CAD build for the part. Positions are in the model's coordinates, mm. Give positions to 0.01 mm unless a question says otherwise; leave off trailing zeros. Loops run counter-clockwise (first coordinate to the right, second up) from the corner with the lowest first, then second, coordinate; pieces in that order, holes last.
Item 1: Probe probe 1 along Z at (x, y) = (-34.5, 0.25); probe 2 along Z at (x, y) = (-27, 0.15); probe 3 along X at (y, z) = (0.3, -26.5). List the from-to ranges inside material, lowest first.
Item 2: Saw through at D-D on z = -15.5. Give the cut face in (x, y), plus the area to 3 significant figures.
Item 3: Saw through at C-C on y = 0.1. Give the number of separate pieces and of enclosed holes in the cut face, plus the area to 3 significant figures.
Item 4: Saw through at B-B on z = -51.5. Give the cut face in (x, y).
Item 5: Saw through at A-A on x = -28.5. Give the cut face in (y, z), plus the area to 3 significant figures.
Autodesk Inventor part; units mm, degrees
ref_plane "YZ Plane" through (0, 0, 0) normal (1, 0, 0) x (0, 1, 0)
ref_plane "XZ Plane" through (0, 0, 0) normal (0, 1, 0) x (-1, 0, 0)
ref_plane "XY Plane" through (0, 0, 0) normal (0, 0, 1) x (1, 0, 0)
sketch "Эскиз1" plane through (0, 0, 0) normal (0, 1, 0) x (-1, 0, 0)
  line L0 (42.275, -3.8) -> (42.275, -4.36)
  arc A0 (40.675, -5.96) -> (42.275, -4.36) centre (40.675, -4.36) ccw
  line L1 (40.675, -5.96) -> (34.325, -5.96)
  arc A1 (32.725, -4.36) -> (34.325, -5.96) centre (34.325, -4.36) ccw
  line L2 (32.725, -4.36) -> (32.725, -3.8)
  arc A2 (34.325, -2.2) -> (32.725, -3.8) centre (34.325, -3.8) ccw
  line L3 (34.325, -2.2) -> (40.675, -2.2)
  arc A3 (42.275, -3.8) -> (40.675, -2.2) centre (40.675, -3.8) ccw
  arc A4 (55.5, -76.631) -> (57.5, -74.631) centre (55.5, -74.631) ccw
  line L4 (55.5, -76.631) -> (19.5, -76.631)
  arc A5 (17.5, -74.631) -> (19.5, -76.631) centre (19.5, -74.631) ccw
  line L5 (17.5, -74.631) -> (17.5, -58.631)
  arc A6 (19.5, -56.631) -> (17.5, -58.631) centre (19.5, -58.631) ccw
  line L6 (19.5, -56.631) -> (55.5, -56.631)
  arc A7 (57.5, -58.631) -> (55.5, -56.631) centre (55.5, -58.631) ccw
  line L7 (57.5, -58.631) -> (57.5, -74.631)
  line L8 (77.5, -85.631) -> (75, -85.631)
  line L9 (75, -47.631) -> (77.5, -47.631)
  line L10 (75, -47.631) -> (75, 0)
  line L11 (75, 0) -> (0, 0)
  line L12 (0, -47.631) -> (0, 0)
  line L13 (-2.5, -47.631) -> (0, -47.631)
  line L14 (0, -85.631) -> (-2.5, -85.631)
  line L15 (0, -85.631) -> (0, -133.2619)
  line L16 (0, -133.2619) -> (75, -133.2619)
  line L17 (75, -85.631) -> (75, -133.2619)
  line L18 (-0.95, -70.631) -> (-2.5, -70.631)
  line L19 (-2.5, -85.631) -> (-2.5, -70.631)
  line L20 (-2.5, -62.631) -> (-2.5, -47.631)
  line L21 (-2.5, -62.631) -> (-0.95, -62.631)
  line L22 (-0.95, -62.631) -> (-0.95, -63.131)
  line L23 (-4.831, -63.131) -> (-0.95, -63.131)
  line L24 (-4.831, -70.131) -> (-0.95, -70.131)
  line L25 (-0.95, -70.131) -> (-0.95, -70.631)
  arc A8 (-4.831, -63.131) -> (-4.831, -70.131) centre (-4.831, -66.631) ccw
  line L26 (77.5, -70.631) -> (77.5, -85.631)
  line L27 (77.5, -70.631) -> (75.95, -70.631)
  line L28 (75.95, -70.631) -> (75.95, -70.131)
  line L29 (79.831, -70.131) -> (75.95, -70.131)
  arc A9 (79.831, -70.131) -> (79.831, -63.131) centre (79.831, -66.631) ccw
  line L30 (79.831, -63.131) -> (75.95, -63.131)
  line L31 (75.95, -63.131) -> (75.95, -62.631)
  line L32 (75.95, -62.631) -> (77.5, -62.631)
  line L33 (77.5, -47.631) -> (77.5, -62.631)
  arc A10 (55.5, -76.631) -> (57.5, -74.631) centre (55.5, -74.631) ccw
  line L34 (57.5, -74.631) -> (57.5, -58.631)
  arc A11 (57.5, -58.631) -> (55.5, -56.631) centre (55.5, -58.631) ccw
  line L35 (55.5, -56.631) -> (19.5, -56.631)
  arc A12 (19.5, -56.631) -> (17.5, -58.631) centre (19.5, -58.631) ccw
  line L36 (17.5, -58.631) -> (17.5, -74.631)
  arc A13 (17.5, -74.631) -> (19.5, -76.631) centre (19.5, -74.631) ccw
  line L37 (19.5, -76.631) -> (55.5, -76.631)
  circle A14 centre (79.831, -66.631) radius 1
  circle A15 centre (-4.831, -66.631) radius 1
  line L38 (42.275, -4.36) -> (42.275, -3.8)
  arc A16 (42.275, -3.8) -> (40.675, -2.2) centre (40.675, -3.8) ccw
  line L39 (40.675, -2.2) -> (34.325, -2.2)
  arc A17 (34.325, -2.2) -> (32.725, -3.8) centre (34.325, -3.8) ccw
  line L40 (32.725, -3.8) -> (32.725, -4.36)
  arc A18 (32.725, -4.36) -> (34.325, -5.96) centre (34.325, -4.36) ccw
  line L41 (34.325, -5.96) -> (40.675, -5.96)
  arc A19 (40.675, -5.96) -> (42.275, -4.36) centre (40.675, -4.36) ccw
  line L42 (0, 0) -> (0, -47.631)
  line L43 (75, 0) -> (0, 0)
  line L44 (75, -47.631) -> (75, 0)
  line L45 (75, -47.631) -> (77.5, -47.631)
  line L46 (77.5, -62.631) -> (77.5, -47.631)
  line L47 (77.5, -62.631) -> (75.95, -62.631)
  line L48 (75.95, -62.631) -> (75.95, -63.131)
  line L49 (75.95, -63.131) -> (79.831, -63.131)
  arc A20 (79.831, -70.131) -> (79.831, -63.131) centre (79.831, -66.631) ccw
  line L50 (79.831, -70.131) -> (75.95, -70.131)
  line L51 (75.95, -70.131) -> (75.95, -70.631)
  line L52 (75.95, -70.631) -> (77.5, -70.631)
  line L53 (77.5, -85.631) -> (77.5, -70.631)
  line L54 (75, -85.631) -> (77.5, -85.631)
  line L55 (75, -133.2619) -> (75, -85.631)
  line L56 (0, -133.2619) -> (75, -133.2619)
  line L57 (0, -85.631) -> (0, -133.2619)
  line L58 (-2.5, -85.631) -> (0, -85.631)
  line L59 (-2.5, -70.631) -> (-2.5, -85.631)
  line L60 (-2.5, -70.631) -> (-0.95, -70.631)
  line L61 (-0.95, -70.631) -> (-0.95, -70.131)
  line L62 (-4.831, -70.131) -> (-0.95, -70.131)
  arc A21 (-4.831, -63.131) -> (-4.831, -70.131) centre (-4.831, -66.631) ccw
  line L63 (-4.831, -63.131) -> (-0.95, -63.131)
  line L64 (-0.95, -63.131) -> (-0.95, -62.631)
  line L65 (-0.95, -62.631) -> (-2.5, -62.631)
  line L66 (-2.5, -47.631) -> (-2.5, -62.631)
  line L67 (-2.5, -47.631) -> (0, -47.631)
  point P0 (40.675, -5.96)
  point P1 (34.325, -5.96)
  point P2 (34.325, -2.2)
extrude "Выдавливание1" add sketch "Эскиз1" along normal blind 0.5
properties part number "metal_body_forPrint"
Results below:
1. probe 1: z = -133.26 to -76.63, -56.63 to -5.96, -2.2 to 0
1. probe 2: z = -133.26 to -76.63, -56.63 to 0
1. probe 3: x = -75 to 0
2. outline: (-75, 0) - (0, 0) - (0, 0.5) - (-75, 0.5) - close
2. area: 37.5 mm2
3. separate pieces: 1
3. enclosed holes: 4
3. area: 9,420 mm2
4. outline: (-77.5, 0) - (2.5, 0) - (2.5, 0.5) - (-77.5, 0.5) - close
5. outline: (0, -133.26) - (0.5, -133.26) - (0.5, -76.63) - (0, -76.63) - close; (0, -56.63) - (0.5, -56.63) - (0.5, 0) - (0, 0) - close
5. area: 56.6 mm2
